Could you check a few things on this model? Use its own coordinates, in mm. A direction names the side the tool comes from. Coordinates: 2 decimals unless noted, no trailing zeros. Order: outer loops, then holes, each group sorted by start corner. A loop starts at its lowest first (then second) coordinate and runs counter-clockwise, first axis right, second up. Notation, with made-up numbers: (61, 86.25) - (100, 86.25) arc R34 cw to (100, 120.25) - close; hole circle Ø5 at (18, 3). An arc over 180 degrees is marked (long way). Answer as CSV lines item,"result". Start each with the question number.
1. I want a section at A-A, the plane y = 44. List the corners of the cut face in (x, z) for me.
2. For faces 1 (the face through (-2.23, 79.99, -2.9)), 2 (the face through (0, 82.88, 0)), which set-ups out of +Z, -Z, +X, -X, +Y, -Y let a thin tool reach every point of the face, with its end or its side?
3. I need wall thicknesses on probe 1 along X at (y, z) = (37, -0.5); probe 2 along Z at (x, y) = (6.25, 39.5); probe 3 along Y at (x, z) = (-7.25, -4.5). Which ranges of each line are inside material? Lowest first, please.
4. For pin 1 (6 mm diameter, centred on y = 36.5, z = 4.5, fed in from +X); pin 2 (2 mm diameter, centred on x = -5, y = 14.5, fed in from +Z); pin 3 (3 mm diameter, centred on y = 36.5, z = -2.5, fed in from -X), each with a flat end and sliding along its axis, tell me the tip position at first contact or that it passes through.
from build123d import *

# Parameters (mm, degrees)
SKETCH2_R           = 9.3218
BOSS_EXTRUDE1_DEPTH = 82.8802
FILLET1_R           = 9.3218
CUT_EXTRUDE1_START  = -13.0302
SKETCH3_R           = 9.3218
SKETCH3_R_2         = 3.6576
CUT_EXTRUDE1_DEPTH  = 13.0302
FILLET2_R           = 9.3218
FILLET3_R           = 5.08
FILLET5_R           = 1.27


with BuildPart() as part:
    # Sketch2 → Boss-Extrude1 (new body)
    with BuildSketch(Plane(origin=(0, 0, 0), x_dir=(1, 0, 0), z_dir=(0, 1, 0))):
        with Locations(Location((0, 0, 0), (0, 0, 270))):
            Circle(SKETCH2_R)
    extrude(amount=BOSS_EXTRUDE1_DEPTH)

    # Fillet1
    fillet1_edges = [part.edges().sort_by_distance(p)[0] for p in [
        (0, 0, -9.3218),
    ]]
    fillet(fillet1_edges, radius=FILLET1_R)

    # Sketch3 → Cut-Extrude1 (cut)
    with BuildSketch(Plane(origin=(0, 82.8802, 0), x_dir=(1, 0, 0), z_dir=(0, 1, 0)).offset(CUT_EXTRUDE1_START)):
        with Locations(Location((0, 0, 0), (0, 0, 90))):
            Circle(SKETCH3_R)
        with Locations(Location((0, 0, 0), (0, 0, 270))):
            Circle(SKETCH3_R_2, mode=Mode.SUBTRACT)
    extrude(amount=CUT_EXTRUDE1_DEPTH, mode=Mode.SUBTRACT)

    # Fillet2
    # the kernel refuses this fillet: 9.3218 mm, written as the material it adds along each edge
    with BuildSketch(Plane(origin=(0, 69.85, 0), x_dir=(0, 0, 1), z_dir=(-1, 0, 0))) as fillet2_piece_1:
        with BuildLine():
            CenterArc((12.9794, 8.574259005), FILLET2_R, 180, 66.897916031)
            Line((3.6576, 8.574259005), (3.471164, 8.574259005))
            Line((3.471164, 8.574259005), (3.471164, 0))
            Line((3.471164, 0), (3.6576, -0.186436))
            ThreePointArc((3.6576, -0.186436), (6.4897, -0.186436), (9.248648, -0.17148518))
            Line((9.248648, -0.17148518), (9.3218, 0))
        make_face()
    revolve(axis=Axis((0, 69.85, 0), (0, 1, 0)))

    # Fillet3
    fillet3_edges = [part.edges().sort_by_distance(p)[0] for p in [
        (0, 69.85, -9.3218),
    ]]
    fillet(fillet3_edges, radius=FILLET3_R)

    # Fillet5
    fillet5_edges = [part.edges().sort_by_distance(p)[0] for p in [
        (0, 82.8802, -3.6576),
    ]]
    fillet(fillet5_edges, radius=FILLET5_R)


solid = part.part
Solved:
1,outline,"circle Ø18.64 at (0, 0)"
2,face 1,"+Y"
2,face 2,"+Z, -Z, +X, -X, +Y"
3,probe 1,"x = -9.31 to 9.31"
3,probe 2,"z = -6.92 to 6.92"
3,probe 3,"y = 5.57 to 69.69"
4,pin 1,"stops at x = 9.2"
4,pin 2,"stops at z = 8.42"
4,pin 3,"stops at x = -9.27"
